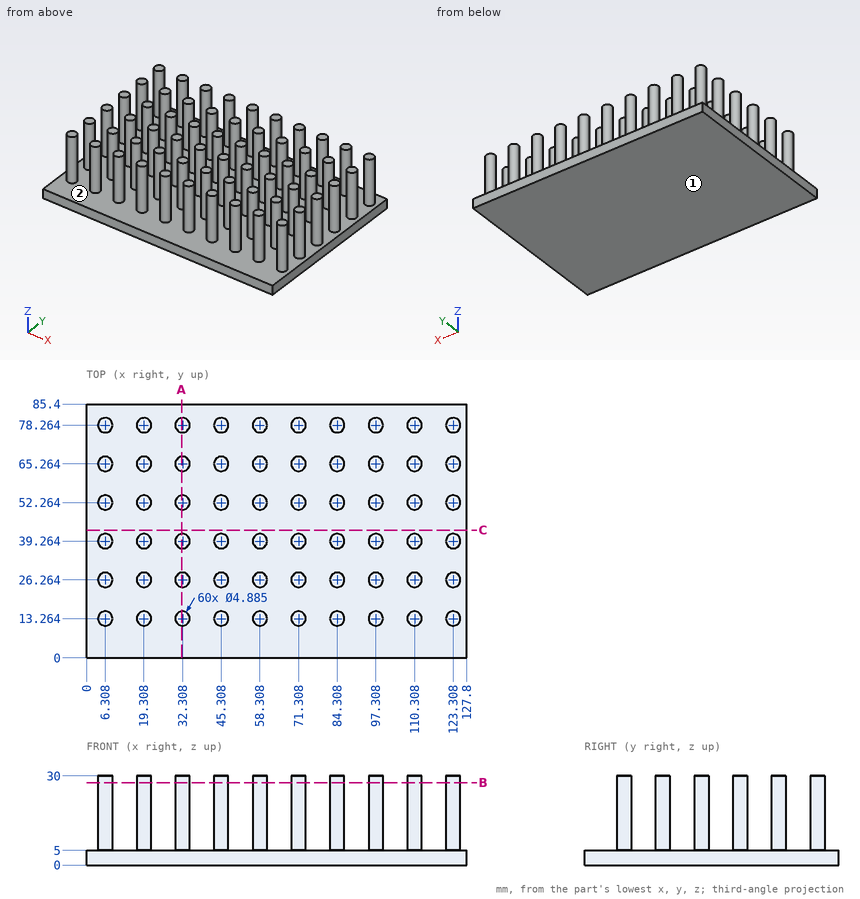
Study the drawing (mm; zero at the part's minimum x, y, z) and answer. Coordinates: 2 decimals unless noted, no trailing zeros. Loops run counter-clockwise (first coordinate to the right, second up) from the corner with the lowest first, then second, coordinate; pieces in that order, holes last. Notation, with made-up numbers: M 36.25,54 L 57.25,54 A24 ccw 57.25,79 Z; hole C 16,-37 d9. An arc over 180 degrees is marked long. Answer in a Markdown table with one row per item. Add a question column.
1. The mould has two halves that part along X. Classify the marked faces 1 and 2: pulls with the +X half, pulls with the -X half, needs draft (parallel to the pull), parting line crosses it, or undercut.
2. Find section C-C, the plane y = 43. Write down the section's boundary in (x, z).
3. Flat-ended cylindrical pins translate along their axes: P1, Ø4, axis at x = 84, z = 22.5, coming from the +Y side; P2, Ø12, axis at y = 64, z = 18.5, coming from the +X side; P3, Ø8, axis at y = 63.5, z = 18, coming from the -X side (1 decimal). Find the tip coordinate at first contact, or state that the pin passes through.
4. Consider L1, parallel to Y at x = 110, z = 8.75; L2, parallel to Y at x = 86.5, z = 5.25 (1 decimal); L3, parallel to Z at x = 66.5, y = 17. Determine where each line is inside the solid, lowest interval first.
5. Find section A-A, the plane x = 32. Write down the section's boundary in (y, z).
6. Find section B-B, the plane z = 27.75. State how many separate pieces and enclosed holes the cut face has.
Reported:
| question | item | result |
|---|---|---|
| 1 | face 1 | needs draft |
| 1 | face 2 | undercut |
| 2 | outline | M 0,0 L 127.8,0 L 127.8,5 L 0,5 Z |
| 3 | P1 | stops at y = 80.71 |
| 3 | P2 | stops at x = 125.75 |
| 3 | P3 | stops at x = 3.9 |
| 4 | L1 | y = 10.84 to 15.69, 23.84 to 28.69, 36.84 to 41.69, 49.84 to 54.69, 62.84 to 67.69, 75.84 to 80.69 |
| 4 | L2 | y = 12.2 to 14.3, 25.2 to 27.3, 38.2 to 40.3, 51.2 to 53.3, 64.2 to 66.3, 77.2 to 79.3 |
| 4 | L3 | z = 0 to 5 |
| 5 | outline | M 0,0 L 85.4,0 L 85.4,5 L 80.69,5 L 80.69,30 L 75.84,30 L 75.84,5 L 67.69,5 L 67.69,30 L 62.84,30 L 62.84,5 L 54.69,5 L 54.69,30 L 49.84,30 L 49.84,5 L 41.69,5 L 41.69,30 L 36.84,30 L 36.84,5 L 28.69,5 L 28.69,30 L 23.84,30 L 23.84,5 L 15.69,5 L 15.69,30 L 10.84,30 L 10.84,5 L 0,5 Z |
| 6 | separate pieces | 60 |
| 6 | enclosed holes | 0 |
